Can you work these out from the model? Positions are in its coordinate system, mm. Face numbers are marked on the shaded views. A direction names the side the tool comes from. Round coordinates to 2 decimals unless told otherwise and drop trailing zeros. Order: outer loops, then holes, each group sorted by start corner. A loop starts at its lowest first (then second) coordinate and runs counter-clockwise, first axis right, second up. Notation, with made-up numbers: (58, 16.5) - (93, 16.5) arc R29 ccw to (93, 54.5) - close; hole circle Ø10 at (-2.5, 25.5). An arc over 180 degrees is marked (long way). Write item = value, one per line.
from build123d import *

# Parameters (mm, degrees)
F1_DEPTH      = 30
F3_DEPTH      = 12.0510542326
F3_DEPTH_BACK = 11.3682544958
F4_SIZE       = 5


with BuildPart() as f1:
    # F0 (on Top) → F1 (new body)
    with BuildSketch(Plane.XY):
        Polygon((-1.1047931817, -12.3112077606), (11.3672544958, -4.8550931739), (8.1301428189, 9.3105951606), (-6.3425499004, 10.6093574387), (-12.0500542326, -2.7536516647), align=None)
    extrude(amount=F1_DEPTH)

    # F2 (on Right) → F3 (cut, two sides)
    with BuildSketch(Plane.YZ) as f3_sk:
        Polygon((0, 21.3343687356), (-7.8424783424, 5.5425534956), (5.5912830867, 5.5425534956), align=None)
    extrude(amount=-F3_DEPTH, mode=Mode.SUBTRACT)
    extrude(f3_sk.sketch, amount=F3_DEPTH_BACK, mode=Mode.SUBTRACT)

    # F4
    f4_edges = [f1.edges().sort_by_distance(p)[0] for p in [
        (9.748699, 2.227751, 30),
    ]]
    chamfer(f4_edges, length=F4_SIZE)


solid = f1.part
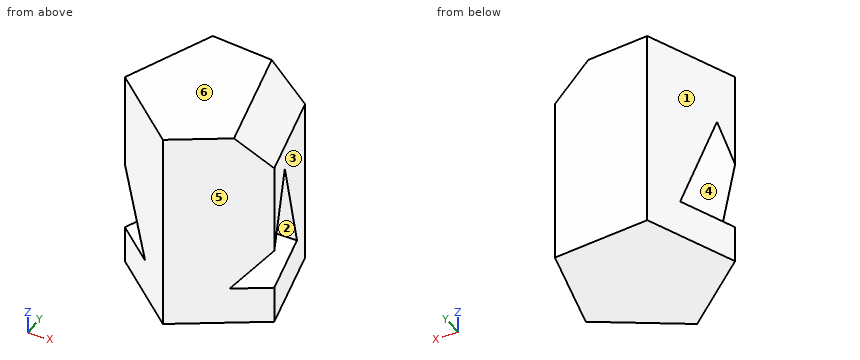
(1) If I drill on line 1 (Z direction, x = 0, y = -5.5); line 2 (Y direction, x = 5.5, z = 6); line 3 (Z direction, x = -0.5, y = -4.25), over which ranges is the centre line in solid material (lowest first)? Write a range as from..to.
Computed:
line_1 = 0..5.54, 10.26..30
line_2 = -8.36..-7.62, 5.43..9.55
line_3 = 0..5.54, 12.78..30
(2) If we section it at C-C (z = 7): Write out the boundary of the cut face in (x, y), plus the area to 3 significant figures.
Computed:
outline = (-8.71, 5.08) - (9.1, 5.08) - (8.13, 9.31) - (-6.34, 10.61) - close; (-7.05, -7.12) - (-1.1, -12.31) - (7.58, -7.12) - close
area = 117 mm^2
(3) If we section it at D-D (x = -5.75): Write out the boundary of the cut face in (y, z), plus the area to 3 significant figures.
Computed:
outline = (-8.25, 0) - (10.56, 0) - (10.56, 30) - (-8.25, 30) - close; hole (-7.84, 5.54) - (5.59, 5.54) - (0, 21.33) - close
area = 458 mm^2
(4) On a 3-axis mill with a long thin cutter (end or side, diameter ignored), from which of +Z, -Z, +X, -X, +Y, -Y can I reach the whole of each face in a straight line? I mean the marked faces 1 and 2. Say none if no direction works.
Computed:
face_1 = +Z, -Z, -X, +Y
face_2 = +X, -X
(5) Will these pins go through, and if not, where does the flat tip stop? P1, Ø4, axis at y = 4, z = 9, coming from the +X side; P2, Ø1, axis at x = 7, y = 0, coming from the -Z side; P3, Ø5, axis at x = 4.5, z = 9.5, coming from the +Y side; P4, Ø1.5, axis at x = 8.5, z = 5.5, coming from the +Y side.
Computed:
P1 = 9.42
P2 = 0
P3 = 9.86
P4 = 9.34
(6) If we section it at B-B (x = -9.5): Write out the boundary of the cut face in (y, z), plus the area to 3 significant figures.
Computed:
outline = (-4.98, 0) - (3.22, 0) - (3.22, 5.54) - (-4.98, 5.54) - close; (-4.98, 11.31) - (0, 21.33) - (3.22, 12.25) - (3.22, 30) - (-4.98, 30) - close
area = 156 mm^2
(7) If we section it at A-A (y = 5): Write out the boundary of the cut face in (x, z).
Computed:
outline = (-8.74, 0) - (9.12, 0) - (9.12, 5.54) - (-8.74, 5.54) - close; (-8.74, 7.21) - (9.12, 7.21) - (9.12, 25) - (3.99, 30) - (-8.74, 30) - close
(8) Thinking about a two-plate mould opening in Y: for the marked faces 3, 4, 5 and 6, which applies, +Y half, -Y half, draft (parallel to the pull), parting line (faces both ways), or undercut?
Computed:
face_3 = +Y half
face_4 = undercut
face_5 = -Y half
face_6 = draft
